Design review of the part shown in the three views and the two pictorial views. Dimensions are in mm from the part's minimum x, y and z. A direction names the side the tool comes from. Give positions to 0.01 mm unless a question says otherwise; leave off trailing zeros. Loops run counter-clockwise (first coordinate to the right, second up) from the corner with the lowest first, then second, coordinate; pieces in that order, holes last. Notation, with made-up numbers: (66, -9.75) -> (122, -9.75) arc R31 cw to (122, 29.25) -> close; hole circle Ø6 at (83.5, -1). An arc over 180 degrees is marked (long way). Answer as CSV lines item,"result".
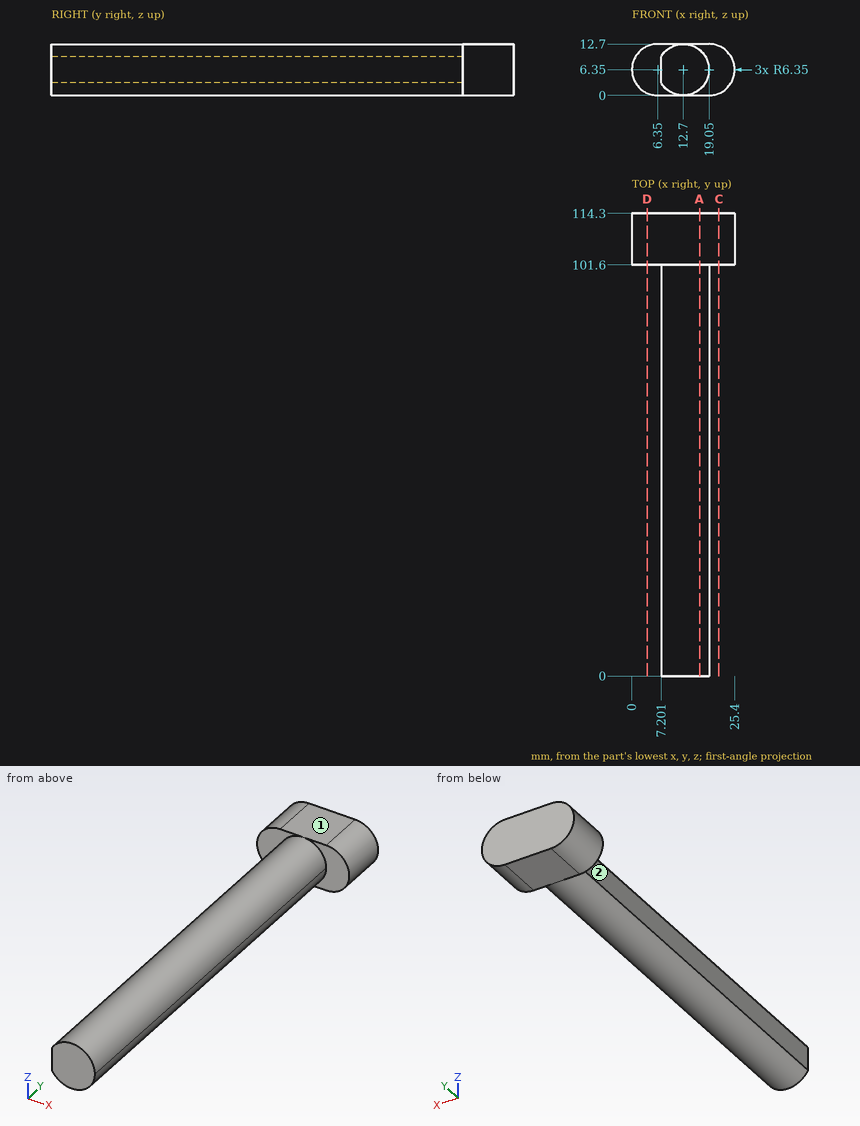
Q1. For the marked faces 1 and 2, list the 3-axis set-ups (+Z, -Z, +X, -X, +Y, -Y) from which the entire face can be reached by the end or side of a thin tool; tool diameter is ignored.
Filled sheet:
face 1,"+Z, +X, -X, +Y, -Y"
face 2,"+Z, -Z, -X, -Y"
Q2. We need section A-A, the plane x = 16.75. State the section outline as (y, z) points, and give its area (4 significant figures).
Filled sheet:
outline,"(0, 1.46) -> (101.6, 1.46) -> (101.6, 0) -> (114.3, 0) -> (114.3, 12.7) -> (101.6, 12.7) -> (101.6, 11.24) -> (0, 11.24) -> close"
area,"1,155 mm^2"
Q3. We need section C-C, the plane x = 21.5. State the section outline as (y, z) points.
Filled sheet:
outline,"(101.6, 0.49) -> (114.3, 0.49) -> (114.3, 12.21) -> (101.6, 12.21) -> close"
Q4. To check wall thickness, follow probe 1 along Z at (x, y) = (12.25, 10.5); probe 2 along Y at (x, z) = (21.5, 1); probe 3 along X at (y, z) = (57.5, 6.25). State the ranges of each line that lie inside material, in increasing order. Write a range as from..to.
Filled sheet:
probe 1,"z = 0.02..12.68"
probe 2,"y = 101.6..114.3"
probe 3,"x = 7.2..19.05"
Q5. We need section D-D, the plane x = 3.75. State the section outline as (y, z) points.
Filled sheet:
outline,"(101.6, 0.56) -> (114.3, 0.56) -> (114.3, 12.14) -> (101.6, 12.14) -> close"
Q6. Clearance check with flat-ended pins moving along their axes: pin 1 Ø3 at (x, y) = (18.5, 34.5) entering from -Z; pin 2 Ø4 at (x, y) = (9, 67) entering from -Z; pin 3 Ø6 at (x, y) = (3.5, 14) entering from +Z; pin 4 Ø2 at (y, z) = (49.5, 8.5) entering from -X. State where each tip first meets the part, or that it passes through.
Filled sheet:
pin 1,"stops at z = 1.68"
pin 2,"stops at z = 0.23"
pin 3,"passes through"
pin 4,"stops at x = 7.2"
